Could you check a few things on this model? Use its own coordinates, in mm. A direction names the side the tool comes from. Round coordinates to 2 decimals unless told otherwise and drop trailing zeros. Loops run counter-clockwise (first coordinate to the right, second up) from the corner with the lowest first, then second, coordinate; pieces in that order, holes last.
from build123d import *

# Parameters (mm, degrees)
F0_W     = 127
F0_H     = 50.8
F1_DEPTH = 76.2
F2_W     = 25.4
F2_H     = 12.7
F3_DEPTH = 76.2
F5_DEPTH = 76.2
F7_DEPTH = 127


with BuildPart() as f1:
    # F0 (on Front) → F1 (new body)
    with BuildSketch(Plane.XZ):
        with Locations((63.5, 25.4)):
            Rectangle(F0_W, F0_H)
    extrude(amount=F1_DEPTH)

    # F2 (on face) → F3 (cut)
    with BuildSketch(Plane.XZ.offset(76.2)):
        Polygon((12.7, 38.1), (12.7, 25.4), (63.5, 25.4), (63.5, 38.1), (50.8, 38.1), (25.4, 38.1), align=None)
        with Locations((38.1, 44.45)):
            Rectangle(F2_W, F2_H)
    extrude(amount=-F3_DEPTH, mode=Mode.SUBTRACT)

    # F4 (on face) → F5 (cut)
    with BuildSketch(Plane.XZ.offset(76.2)):
        Polygon((127, 50.8), (76.2, 50.8), (82.55, 38.1), (127, 38.1), align=None)
    extrude(amount=-F5_DEPTH, mode=Mode.SUBTRACT)

    # F6 (on face) → F7 (cut)
    with BuildSketch(Plane.YZ.offset(127)):
        Polygon((-57.15, 12.7), (-76.2, 12.7), (-76.2, 0), (-63.5, 0), align=None)
        Polygon((0, 0), (0, 12.7), (-19.05, 12.7), (-12.7, 0), align=None)
    extrude(amount=-F7_DEPTH, mode=Mode.SUBTRACT)


solid = f1.part
Item 1: If I drill on line 1 along Z through (x, y) = (14, -48); line 2 along X through (y, z) = (-15.5, 27); line 3 along Z through (x, y) = (86.5, -21.5), over which ranges is the centre line in solid material (lowest first)?
Results list:
line 1: z = 0 to 25.4, 38.1 to 50.8
line 2: x = 0 to 12.7, 63.5 to 127
line 3: z = 0 to 38.1
Item 2: If we section it at C-C, the plane x = 34: Please give me the cut outline in (y, z).
Results list:
outline: (-76.2, 12.7) - (-57.15, 12.7) - (-63.5, 0) - (-12.7, 0) - (-19.05, 12.7) - (0, 12.7) - (0, 25.4) - (-76.2, 25.4) - close
Item 3: Will these pins go through, and if not, where does the flat tip stop? pin 1 (6.5 mm diameter, centred on y = -27, z = 42.5, fed in from +X) (3 decimals); pin 2 (1 mm diameter, centred on x = 35.5, y = -52.5, fed in from +Z); pin 3 (4 mm diameter, centred on x = 79, y = -68, fed in from -Z).
Results list:
pin 1: stops at x = 81.975
pin 2: stops at z = 25.4
pin 3: stops at z = 12.7
Item 4: If we section it at D-D, the plane y = -37: Please give me the cut outline in (x, z), then the cut area to 3 significant figures.
Results list:
outline: (0, 0) - (127, 0) - (127, 38.1) - (82.55, 38.1) - (76.2, 50.8) - (50.8, 50.8) - (50.8, 38.1) - (63.5, 38.1) - (63.5, 25.4) - (12.7, 25.4) - (12.7, 38.1) - (25.4, 38.1) - (25.4, 50.8) - (0, 50.8) - close
area: 4,880 mm2
Item 5: If we section it at B-B, the plane x = 58.5: Please give me the cut outline in (y, z), then the cut area to 3 significant figures.
Results list:
outline: (-76.2, 12.7) - (-57.15, 12.7) - (-63.5, 0) - (-12.7, 0) - (-19.05, 12.7) - (0, 12.7) - (0, 25.4) - (-76.2, 25.4) - close; (-76.2, 38.1) - (0, 38.1) - (0, 50.8) - (-76.2, 50.8) - close
area: 2,500 mm2
Item 6: If we section it at A-A, the plane z = 40.5: Please give me the cut outline in (x, y), then the cut area to 3 significant figures.
Results list:
outline: (0, -76.2) - (25.4, -76.2) - (25.4, 0) - (0, 0) - close; (50.8, -76.2) - (81.35, -76.2) - (81.35, 0) - (50.8, 0) - close
area: 4,260 mm2
Item 7: For faces 4 (the flat face through (64.39, -60.37, 6.26)), 5 (the flat face through (64, -9, 12.7)), 6 (the flat face through (38, -39, 25.4)), 7 (the flat face through (25.4, -39, 44)), 8 (the flat face through (104, -39, 38.1)), which set-ups out of +Z, -Z, +X, -X, +Y, -Y let a thin tool reach every point of the face, with its end or its side?
Results list:
face 4: +X, -X, -Y
face 5: +X, -X, +Y
face 6: +Y, -Y
face 7: +Z, +Y, -Y
face 8: +Z, +X, +Y, -Y
Item 8: We'd pull the mould along X, two halves only. Please class faces 1 (the flat face through (63.5, -39, 32)), 2 (the flat face through (64, -67, 12.7)), 3 (the flat face through (79.33, -38.63, 44.54)): released by +X, released by -X, zero draft, split by the parting line, or undercut.
Results list:
face 1: undercut
face 2: zero draft
face 3: released by +X
